Part model, mm, in its own coordinate system. A direction names the side the tool comes from. Round coordinates to 2 decimals unless told otherwise and drop trailing zeros. Write each loop counter-clockwise with the first axis right and the second up, starting at its lowest first coordinate (ties: lowest second). Pieces come first, ordered by that corner, then holes. Notation, with made-up numbers: M 9,54.25 L 43,54.25 A13 cw 43,79.25 Z; hole C -14.5,69.5 d7. An arc over 180 degrees is marked long. One line per question, with ' | ' between items. Start each with the question number.
1) Drop flat-ended pins along their axis: pin 1 Ø5 at (x, y) = (-36.5, -4.5) entering from -Z; pin 2 Ø5.5 at (x, y) = (-24.5, -13) entering from +Z; pin 3 Ø5 at (x, y) = (-32.5, -13) entering from -Z; pin 4 Ø7 at (x, z) = (-11.27, 43.99) entering from -Y. Give the stop position or say it passes through.
2) Saw through at D-D (x = 6). List the corners of the cut face in (y, z), plus the area to 3 significant figures.
3) Saw through at A-A (y = -13.5). List the corners of the cut face in (x, z), plus the area to 3 significant figures.
4) Saw through at B-B (x = -12). List the corners of the cut face in (y, z).
5) Tool access for faces 5 (the face through (-25, -12, 19.063)), 6 (the face through (-10, -12, 11.731)), 7 (the face through (-35.7, -12.5, 40.2)), 8 (the face through (-4.491, -12, 10)), 9 (the face through (-49.949, -5, 24)): list every direction of +Z, -Z, +X, -X, +Y, -Y with a clear straight run to the whole face (end or side of a thin tool).
6) Wall check: probe 1 along Y at (x, z) = (-45, 1); probe 2 along Z at (x, y) = (12.5, -10.75); probe 3 along Z at (x, y) = (-8, -2.25). Give the ranges that are in metal, low to high. Write a range as [from, to].
7) Saw through at C-C (y = -1.5). List the corners of the cut face in (x, z), plus the area to 3 significant figures.
8) Mould opens along X. For faces 1 (the face through (6.808, -12.465, 20.758)), 2 (the face through (31.398, -5.07, 0.122)), 3 (the face through (-49.46, -5.07, 0.27)), 4 (the face through (-15.122, -12, 10)) say: pulls with the +X half, pulls with the -X half, needs draft (parallel to the pull), parting line crosses it, or undercut.
```python
from build123d import *

# Parameters (mm, degrees)
F1_DEPTH = 10
F2_W     = 10.631341
F2_H     = 4.399176
F3_DEPTH = 5
F4_R     = 3.948378
F5_DEPTH = 101.092
F6_R     = 5.08


with BuildPart() as f1:
    # F0 (on Front) → F1 (new body)
    with BuildSketch(Plane.XZ):
        Polygon((31.674738, 50.957117), (-49.948968, 50.957117), (-49.948968, 0), (0, -39.775878), (31.674738, 0), align=None)
    extrude(amount=F1_DEPTH)

    # F2 (on face) → F3 (join)
    with BuildSketch(Plane.XZ.offset(10)):
        Polygon((-37.851237, 24.562063), (-30.15268, 47.657736), (-41.333918, 32.627217), (-41.333918, 3.299381), (-15.855361, 19.063093), (-34.735154, 19.063093), (-30.519279, 15.213814), (-36.257481, 8.929118), align=None)
        Polygon((7.973504, 34.826804), (23.920517, 47.657736), (0, 38.859382), (-4.490824, 19.063093), (7.183906, 10.378234), (22.454122, 19.063093), (9.439895, 16.13031), (4.101735, 25.516167), align=None)
        with Locations((-9.806494, 9.531547)):
            Rectangle(F2_W, F2_H)
    extrude(amount=F3_DEPTH)

    # F4 (on face) → F5 (cut)
    with BuildSketch(Plane.XZ.offset(10)):
        with Locations((-11.272887, 43.991752)):
            Circle(F4_R)
    extrude(amount=-F5_DEPTH, mode=Mode.SUBTRACT)

    # F6
    f6_edges = [f1.edges().sort_by_distance(p)[0] for p in [
        (-49.948968, -5, 50.957117),
        (31.674738, -5, 50.957117),
        (31.674738, -5, 0),
        (0, -5, -39.775878),
        (-49.948968, -5, 0),
    ]]
    fillet(f6_edges, radius=F6_R)


solid = f1.part
```
Answer key:
1) pin 1: stops at z = -12.7 | pin 2: stops at z = 19.06 | pin 3: stops at z = 7.22 | pin 4: passes through
2) outline: M -15,11.26 L -10,11.26 L -10,-32.24 L 0,-32.24 L 0,50.96 L -10,50.96 L -10,41.07 L -15,41.07 L -15,30.08 L -10,30.08 L -10,22.18 L -15,22.18 Z | area: 942 mm2
3) outline: M -41.33,3.3 L -15.86,19.06 L -34.74,19.06 L -30.52,15.21 L -36.26,8.93 L -37.85,24.56 L -30.15,47.66 L -41.33,32.63 Z; M -15.12,7.33 L -4.49,7.33 L -4.49,11.73 L -15.12,11.73 Z; M -4.49,19.06 L 7.18,10.38 L 22.45,19.06 L 9.44,16.13 L 4.1,25.52 L 7.97,34.83 L 23.92,47.66 L 0,38.86 Z | area: 650 mm2
4) outline: M -15,7.33 L -10,7.33 L -10,-30.22 L 0,-30.22 L 0,40.11 L -10,40.11 L -10,11.73 L -15,11.73 Z; M -10,47.87 L 0,47.87 L 0,50.96 L -10,50.96 Z
5) face 5: -Y | face 6: +Z, -Y | face 7: +Z, -X, -Y | face 8: -Z, -Y | face 9: +Z, -Z, -X, +Y, -Y
6) probe 1: y = [-10, 0] | probe 2: z = [13.4, 16.82], [38.47, 43.46] | probe 3: z = [-33.41, 41.78], [46.2, 50.96]
7) outline: M -49.95,2.45 A5.08 ccw -48.03,-1.53 L -3.97,-36.61 A5.08 ccw 3.16,-35.8 L 30.57,-1.39 A5.08 ccw 31.67,1.78 L 31.67,45.88 A5.08 ccw 26.59,50.96 L -44.87,50.96 A5.08 ccw -49.95,45.88 Z; hole C -11.27,43.99 d7.9 | area: 5,720 mm2
8) face 1: undercut | face 2: pulls with the +X half | face 3: pulls with the -X half | face 4: undercut
